Source: CAD feature listing. Evaluate the final solid. Frame: model axes, mm. Round coordinates to 2 decimals unless told otherwise and drop trailing zeros. Order: outer loops, then holes, each group sorted by start corner. A loop starts at its lowest first (then second) coordinate and runs counter-clockwise, first axis right, second up. Notation, with made-up numbers: (16, 32.5) - (63, 32.5) arc R23 cw to (63, 71.5) - close; hole circle Ø7 at (52, 55.5). An arc over 180 degrees is marked (long way). Return JSON: item names as keys, results as strings. Group by question number.
1) Section B-B, the plane x = 0.8. Give the number of separate pieces and of enclosed holes in the cut face, plus the area to 3 significant figures.
2) Section D-D, the plane y = 26. Return loops of the section in (x, z), plus the area to 3 significant figures.
3) Contact query for flat-ended pins moving along their axis: P1, Ø2.5, axis at y = -9, z = 0, coming from the -X side; P2, Ø2.5, axis at y = 26, z = 7, coming from the -X side; P3, Ø4, axis at y = 2, z = 29, coming from the +X side; P4, Ø0.8, axis at x = 0.5, z = -0.5, coming from the -Y side. Output: stop coordinate, or through.
4) Section C-C, the plane z = 13. Return loops of the section in (x, y).
5) Ray query, line 1 (Z direction, x = 0.15, y = -5.5); line 2 (Z direction, x = 0.1, y = 2); line 3 (Y direction, x = 1.2, z = 9). Return the intervals inside material, ascending. Write a range as from..to.
6) Section A-A, the plane y = -6. Return loops of the section in (x, z).
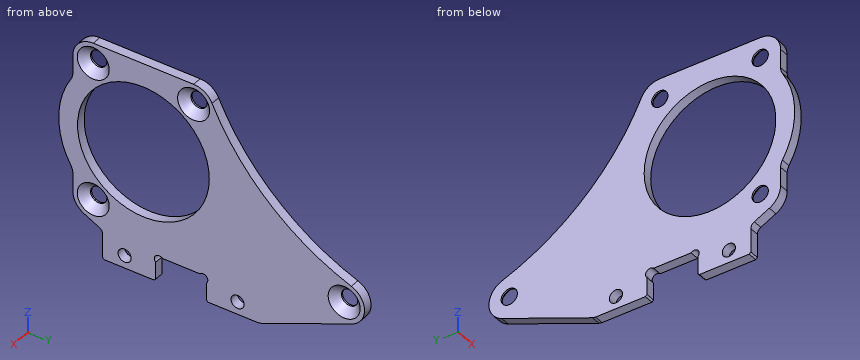
Autodesk Inventor part; units mm, degrees
ref_plane "YZ Plane" through (0, 0, 0) normal (1, 0, 0) x (0, 1, 0)
ref_plane "XZ Plane" through (0, 0, 0) normal (0, 1, 0) x (-1, 0, 0)
ref_plane "XY Plane" through (0, 0, 0) normal (0, 0, 1) x (1, 0, 0)
sketch "スケッチ1" plane through (0, 0, 0) normal (1, 0, 0) x (0, 1, 0)
  line L0 (12.5, 2) -> (-12.5, 2) construction
  line L1 (-12.5, 2) -> (-12.5, -2)
  line L2 (-12.5, -2) -> (-4.05, -2)
  line L3 (12.5, -2) -> (12.5, 2) construction
  line L4 (0, 0) -> (0, 21.2341) construction
  line L5 (0, 0) -> (25.6299, 0) construction
  circle A0 centre (9, 0) radius 1.05
  circle A1 centre (-9, 0) radius 1.05
  line L6 (-17.25, 7) -> (-17.25, 9.9571)
  line L7 (-14, 32.25) -> (2, 32.25)
  arc A2 (4.9363, 30.393) -> (27.1329, 10.0462) centre (41.0759, 47.5374) ccw
  arc A3 (-17.25, 7) -> (-15.4518, 4.0923) centre (-14, 7) ccw
  arc A4 (-14, 32.25) -> (-17.25, 29) centre (-14, 29) ccw
  arc A5 (4.9363, 30.393) -> (2, 32.25) centre (2, 29) ccw
  circle A6 centre (2, 29) radius 1.3
  circle A7 centre (-14, 29) radius 1.3
  circle A8 centre (-14, 7) radius 1.3
  circle A9 centre (26, 7) radius 1.3
  arc A10 (27.2246, 3.9895) -> (27.1329, 10.0462) centre (26, 7) ccw
  line L8 (2, 29) -> (-14, 29) construction
  line L9 (-6, 29) -> (-6, 7) construction
  line L10 (-6, 7) -> (-14, 7) construction
  circle A11 centre (-6, 18) radius 10.5
  arc A12 (-17.5403, 25.0051) -> (-17.5403, 10.9949) centre (-6, 18) ccw
  line L11 (-17.25, 10.5376) -> (-17.25, 25.4624) construction
  line L12 (-17.25, 26.0429) -> (-17.25, 29)
  arc A13 (-17.5403, 25.0051) -> (-17.25, 26.0429) centre (-19.25, 26.0429) ccw
  arc A14 (-17.25, 9.9571) -> (-17.5403, 10.9949) centre (-19.25, 9.9571) ccw
  line L13 (-6, 18) -> (10, 18) construction
  line L14 (27.2246, 3.9895) -> (12.5, -2)
  line L15 (-4.05, -2) -> (-4.05, 0.9893)
  line L16 (-4.05, 2.05) -> (-2.9893, 2.05) construction
  line L17 (4.05, 2.05) -> (4.05, 0.9893) construction
  line L18 (-4.05, -2) -> (4.05, -2) construction
  line L19 (4.05, -2) -> (12.5, -2)
  arc A15 (4.05, 0.9893) -> (2.9893, 2.05) centre (3.5197, 1.5197) ccw
  line L20 (4.05, 0.9893) -> (4.05, -2)
  line L21 (2.9893, 2.05) -> (4.05, 2.05) construction
  line L22 (-2.9893, 2.05) -> (2.9893, 2.05)
  line L23 (-4.05, 0.9893) -> (-4.05, 2.05) construction
  arc A16 (-2.9893, 2.05) -> (-4.05, 0.9893) centre (-3.5197, 1.5197) ccw
  line L24 (3.5197, 1.5197) -> (4.05, 2.05) construction
  line L25 (-3.5197, 1.5197) -> (-4.05, 2.05) construction
  line L26 (-12.5, -2) -> (-12.5, 2) construction
  arc A17 (-12.5, 2) -> (-13.0533, 2.8947) centre (-13.5, 2) ccw
  line L27 (-15.4518, 4.0923) -> (-13.0533, 2.8947)
  point P0 (4.1125, 32.25)
  point P1 (16.6739, 3.086)
  dimension "d2" = 18
  dimension "d3" = 2.1
  dimension "d7" = 16
  dimension "d8" = 2.6
  dimension "d13" = 3.25
  dimension "d14" = 21
  dimension "d15" = 40
  dimension "d17" = 40
  dimension "d18" = 6
  dimension "d21" = 3
  dimension "d22" = 2
  dimension "d27" = 18
  dimension "d28" = 22
  dimension "d30" = 8.1
  dimension "d31" = 4
  dimension "d32" = 4.05
  dimension "d33" = 0.75
  dimension "d34" = 45
  dimension "d35" = 45
  dimension "d36" = 1
extrude "押し出し1" add sketch "スケッチ1" along normal blind 1.5
chamfer "面取り1" distance 0.25 angle 45 4 edges at (0.75, -12.5, -2) (0.75, -4.05, -2) (0.75, 4.05, -2) (0.75, 12.5, -2)
chamfer "面取り2" distance 1.25 angle 45 4 edges at (1.5, 24.7, 7) (1.5, 0.7, 29) (1.5, -15.3, 29) (1.5, -15.3, 7)
properties part number "16_006_COXA_FRAME_1_R1"
Geometry check:
{
 "1": {"separate pieces": "1", "enclosed holes": "7", "area": "720 mm2"},
 "2": {"outline": "(0, 3.49) - (1.5, 3.49) - (1.5, 4.45) - (0.25, 5.7) - (0, 5.7) - close; (0, 8.3) - (0.25, 8.3) - (1.5, 9.55) - (1.5, 10.49) - (0, 10.49) - close", "area": "5.03 mm2"},
 "3": {"P1": "x = 0", "P2": "through", "P3": "x = 0.95", "P4": "y = -12.5"},
 "4": {"outline": "(0, -18.54) - (1.5, -18.54) - (1.5, -15.23) - (0, -15.23) - close; (0, 3.23) - (1.5, 3.23) - (1.5, 20.9) - (0, 20.9) - close"},
 "5": {"line 1": "-2..7.51, 28.49..32.25", "line 2": "2.05..11.2, 24.8..27.7, 30.3..32.25", "line 3": "-17.25..-15.03, -12.97..-11.41, -0.59..24.97, 27.03..28.56"},
 "6": {"outline": "(0, -2) - (1.5, -2) - (1.5, 7.5) - (0, 7.5) - close; (0, 28.5) - (1.5, 28.5) - (1.5, 32.25) - (0, 32.25) - close"}
}
